from build123d import *

# Parameters (mm, degrees)
ESQUISSE1_W        = 7
ESQUISSE1_H        = 2.5
BOSS_EXTRU_1_DEPTH = 6.5
ESQUISSE2_R        = 0.25
BOSS_EXTRU_2_DEPTH = 3.6


with BuildPart() as part:
    # Esquisse1 → Boss.-Extru.1 (new body)
    with BuildSketch(Plane.XY):
        Rectangle(ESQUISSE1_W, ESQUISSE1_H)
    extrude(amount=BOSS_EXTRU_1_DEPTH)

    # Esquisse2 → Boss.-Extru.2 (add)
    with BuildSketch(Plane(origin=(0, 0, 0), x_dir=(-1, 0, 0), z_dir=(0, 0, -1))):
        with Locations((-2.5, 0)):
            Circle(ESQUISSE2_R)
        with Locations((2.5, 0)):
            Circle(ESQUISSE2_R)
    extrude(amount=BOSS_EXTRU_2_DEPTH)


solid = part.part
CAD build for the part. Positions are in the model's coordinates, mm. Round coordinates to 2 decimals unless told otherwise and drop trailing zeros. Loops run counter-clockwise (first coordinate to the right, second up) from the corner with the lowest first, then second, coordinate; pieces in that order, holes last.
(1) Cut at C-C (y = -0.6). Give the cut face in (x, z), plus the area to 3 significant figures.
(2) Cut at A-A (x = 2.5). Give the cut face in (y, z).
(3) Wall check: line 1 along Z through (x, y) = (-2.75, 0.45). Give the ranges that are in metal, low to high.
(4) Cut at B-B (z = -1). Give the cut face in (x, y), plus the area to 3 significant figures.
(5) Cut at D-D (x = -1.75). Give the cut face in (y, z), plus the area to 4 significant figures.
Findings below:
1. outline: (-3.5, 0) - (3.5, 0) - (3.5, 6.5) - (-3.5, 6.5) - close
1. area: 45.5 mm2
2. outline: (-1.25, 0) - (-0.25, 0) - (-0.25, -3.6) - (0.25, -3.6) - (0.25, 0) - (1.25, 0) - (1.25, 6.5) - (-1.25, 6.5) - close
3. line 1: z = 0 to 6.5
4. outline: circle Ø0.5 at (-2.5, 0); circle Ø0.5 at (2.5, 0)
4. area: 0.393 mm2
5. outline: (-1.25, 0) - (1.25, 0) - (1.25, 6.5) - (-1.25, 6.5) - close
5. area: 16.25 mm2
